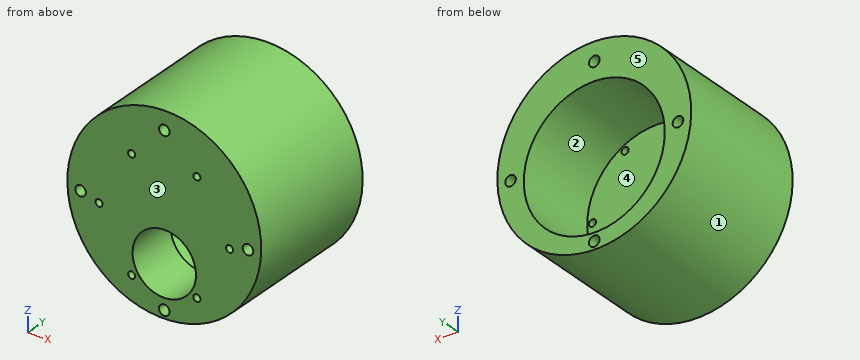
```python
from build123d import *

# Parameters (mm, degrees)
SKETCH1_R                = 27.5
SKETCH1_R_2              = 1
BOSS_EXTRUDE2_DEPTH      = 15
CUT_EXTRUDE17_DEPTH      = 44.720704477
CUT_EXTRUDE17_DEPTH_BACK = 44.720704477
SKETCH2_R                = 9
SKETCH7_R                = 27.5
SKETCH7_R_2              = 20
BOSS_EXTRUDE4_DEPTH      = 25
CUT_EXTRUDE18_DEPTH      = 58.328003628
CUT_EXTRUDE18_DEPTH_BACK = 58.328003628
SKETCH8_R                = 1.5


with BuildPart() as part:
    # Sketch1 → Boss-Extrude2 (new body)
    with BuildSketch(Plane(origin=(0, 0, 0), x_dir=(1, 0, 0), z_dir=(0, 1, 0))):
        with Locations(Location((0, -3, 0), (0, 0, 270))):
            Circle(SKETCH1_R)
        with Locations(Location((9.25, 16.02146997, 0), (0, 0, 270))):
            Circle(SKETCH1_R_2, mode=Mode.SUBTRACT)
        with Locations(Location((18.5, 0, 0), (0, 0, 270))):
            Circle(SKETCH1_R_2, mode=Mode.SUBTRACT)
        with Locations(Location((9.25, -16.02146997, 0), (0, 0, 270))):
            Circle(SKETCH1_R_2, mode=Mode.SUBTRACT)
        with Locations(Location((-9.25, -16.02146997, 0), (0, 0, 270))):
            Circle(SKETCH1_R_2, mode=Mode.SUBTRACT)
        with Locations(Location((-18.5, 0, 0), (0, 0, 270))):
            Circle(SKETCH1_R_2, mode=Mode.SUBTRACT)
        with Locations(Location((-9.25, 16.02146997, 0), (0, 0, 270))):
            Circle(SKETCH1_R_2, mode=Mode.SUBTRACT)
    extrude(amount=BOSS_EXTRUDE2_DEPTH)

    # Sketch2 → Cut-Extrude17 (cut, two sides: drawn at the far end of the back side and taken through both)
    with BuildSketch(Plane(origin=(0, 15, 0), x_dir=(1, 0, 0), z_dir=(0, 1, 0)).offset(-CUT_EXTRUDE17_DEPTH_BACK)):
        with Locations(Location((0, 10, 0), (0, 0, 270))):
            Circle(SKETCH2_R)
    extrude(amount=CUT_EXTRUDE17_DEPTH + CUT_EXTRUDE17_DEPTH_BACK, mode=Mode.SUBTRACT)

    # Sketch7 → Boss-Extrude4 (add)
    with BuildSketch(Plane(origin=(0, 15, 0), x_dir=(1, 0, 0), z_dir=(0, 1, 0))):
        with Locations(Location((0, -3, 0), (0, 0, 270))):
            Circle(SKETCH7_R)
        with Locations(Location((0, 0, 0), (0, 0, 270))):
            Circle(SKETCH7_R_2, mode=Mode.SUBTRACT)
    extrude(amount=BOSS_EXTRUDE4_DEPTH)

    # Sketch8 → Cut-Extrude18 (cut, two sides: drawn at the far end of the back side and taken through both)
    with BuildSketch(Plane(origin=(0, 40, 0), x_dir=(1, 0, 0), z_dir=(0, 1, 0)).offset(-CUT_EXTRUDE18_DEPTH_BACK)):
        with Locations(Location((0, 22.25, 0), (0, 0, 270))):
            Circle(SKETCH8_R)
        with Locations(Location((23.75, -1.5, 0), (0, 0, 270))):
            Circle(SKETCH8_R)
        with Locations(Location((0, -25.25, 0), (0, 0, 270))):
            Circle(SKETCH8_R)
        with Locations(Location((-23.75, -1.5, 0), (0, 0, 270))):
            Circle(SKETCH8_R)
    extrude(amount=CUT_EXTRUDE18_DEPTH + CUT_EXTRUDE18_DEPTH_BACK, mode=Mode.SUBTRACT)


solid = part.part
```
CAD build for the part. Positions are in the model's coordinates, mm. Face numbers are marked on the shaded views. A direction names the side the tool comes from. Coordinates: 2 decimals unless noted, no trailing zeros. Write each loop counter-clockwise with the first axis right and the second up, starting at its lowest first coordinate (ties: lowest second). Pieces come first, ordered by that corner, then holes.
(1) Cut at A-A, the plane y = 12.5. Count the separate pieces of the cut face and the enclosed holes in it, and give its area (3 significant figures).
(2) Cut at B-B, the plane z = 25. List the corners of the cut face in (x, y).
(3) Drill centre lines: probe 1 along X at (y, z) = (32, 1.5); probe 2 along Z at (x, y) = (-1, 37.5); probe 3 along X at (y, z) = (12.5, 2). Where is each one in solid material? Low to high.
(4) Cut at C-C, the plane y = 34.5. List the corners of the cut face in (x, z).
(5) 3-axis set-ups, long thin cutter, end or side, ignore diameter. For the marked faces 4 and 5: which of +Z, -Z, +X, -X, +Y, -Y reach the whole face in a straight line?
(6) Two-plate mould, pull along Z, no slides. Class the marked faces 1, 2 and 3: +Z half, -Z half, draft (parallel to the pull), parting line (faces both ways), or undercut.
(7) Cut at D-D, the plane x = 11. List the corners of the cut face in (y, z).
(8) Flat gauge pins, fed straight in: pin 1 (12 mm diameter, centred on x = 18.5, y = 29.5, fed in from +Z); pin 2 (1.5 mm diameter, centred on x = -5, y = 12.5, fed in from -Z); pin 3 (1.2 mm diameter, centred on x = -18.5, z = 0, fed in from -Y); pin 4 (1.5 mm diameter, centred on x = 3, y = 21.5, fed in from +Z). Where does each tip first touch, or does it go through?
Geometry says:
1. separate pieces: 1
1. enclosed holes: 11
1. area: 2,070 mm2
2. outline: (-16.5, 0) - (-1.48, 0) - (-1.48, 40) - (-16.5, 40) - close; (1.48, 0) - (16.5, 0) - (16.5, 40) - (1.48, 40) - close
3. probe 1: x = -27.46 to -25.25, -22.25 to -19.94, 19.94 to 22.25, 25.25 to 27.46
3. probe 2: z = -24.48 to -23.37, -21.13 to -19.97, 19.97 to 24.13, 26.37 to 30.48
3. probe 3: x = -27.48 to -25.16, -22.34 to 22.34, 25.16 to 27.48
4. outline: circle Ø55 at (0, 3); hole circle Ø3 at (-23.75, 1.5); hole circle Ø40 at (0, 0); hole circle Ø3 at (0, -22.25); hole circle Ø3 at (0, 25.25); hole circle Ø3 at (23.75, 1.5)
5. face 4: +Y
5. face 5: +Z, -Z, +X, -X, +Y
6. face 1: parting line
6. face 2: undercut
6. face 3: draft
7. outline: (0, -22.2) - (40, -22.2) - (40, -16.7) - (15, -16.7) - (15, 16.7) - (40, 16.7) - (40, 28.2) - (0, 28.2) - close
8. pin 1: stops at z = 27.49
8. pin 2: stops at z = -24.17
8. pin 3: passes through
8. pin 4: stops at z = 30.41
